Build history of the part. All positions in model axes, mm. Face numbers are marked on the shaded views. A direction names the side the tool comes from. Give positions to 0.01 mm unless a question says otherwise; leave off trailing zeros. Write each loop counter-clockwise with the first axis right and the second up, starting at its lowest first coordinate (ties: lowest second). Pieces come first, ordered by that corner, then holes. Notation, with made-up numbers: M -3,-4.5 L 16,-4.5 A21 ccw 16,11.5 Z; hole C 28,-9 d5. An arc over 180 degrees is marked long. Return JSON: item names as keys, results as strings. Group by question number.
Q1. Band-saw the part on A-A, the plane y = 1. Give the cut face in (x, z).
Q2. Wall check: probe 1 along Y at (x, z) = (1.4, 5.25); probe 2 along Z at (x, y) = (1.95, 5.25); probe 3 along Z at (x, y) = (0.2, 3). Give the ranges that are in metal, low to high.
Q3. Band-saw the part on B-B, the plane z = 2.75. Give the cut face in (x, y), then the cut area to 3 significant figures.
Q4. Pull direction Z, two halves, no side cores. Call the marked faces 1, 2 and 3: +Z half, -Z half, draft (parallel to the pull), parting line (faces both ways), or undercut.
Q5. Flat gauge pins, fed straight in: pin 1 Ø1.5 at (x, y) = (2, 1) entering from -Z; pin 2 Ø1.5 at (x, y) = (0.5, 0) entering from +Z; pin 3 Ø4 at (y, z) = (0, -0.5) entering from -X. Where does each tip first touch, or does it go through?
Q6. Tool access for the marked faces 4 and 5: list every direction of +Z, -Z, +X, -X, +Y, -Y with a clear straight run to the whole face (end or side of a thin tool).
Q7. Band-saw the part on D-D, the plane y = 13.5. Give the cut face in (x, z).
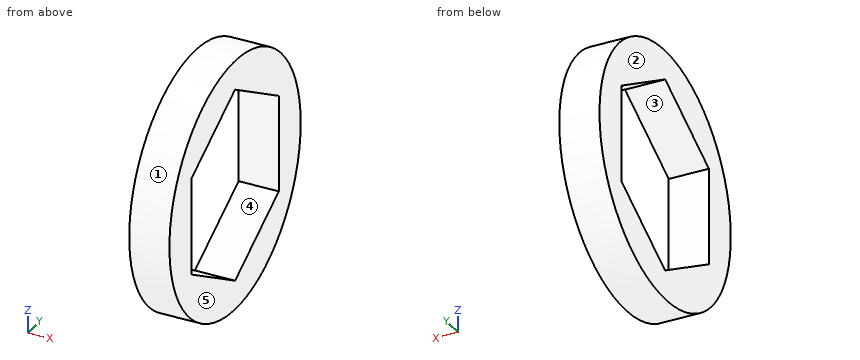
Autodesk Inventor part; units mm, degrees
ref_plane "YZ Plane" through (0, 0, 0) normal (1, 0, 0) x (0, 1, 0)
ref_plane "XZ Plane" through (0, 0, 0) normal (0, 1, 0) x (-1, 0, 0)
ref_plane "XY Plane" through (0, 0, 0) normal (0, 0, 1) x (1, 0, 0)
sketch "Sketch1" plane through (0, 0, 0) normal (1, 0, 0) x (0, 1, 0)
  circle A0 centre (5.9226, 5.0314) radius 9.525
  line L0 (5.9226, 5.0314) -> (12.2726, 5.0314) construction
  line L1 (12.2726, 1.3724) -> (5.9287, -2.2974)
  line L2 (5.9287, -2.2974) -> (-0.4213, 1.3617)
  line L3 (-0.4213, 1.3617) -> (-0.4274, 8.6905)
  line L4 (-0.4274, 8.6905) -> (5.9164, 12.3602)
  line L5 (5.9164, 12.3602) -> (12.2664, 8.7012)
  line L6 (12.2664, 8.7012) -> (12.2726, 1.3724)
  point P0 (0, 0)
  dimension "d0" = 19.05
extrude "Extrusion1" add sketch "Sketch1" along normal blind 3.0226
properties part number "3D Model Spacer"
From the geometry:
{
 "1": {"outline": "M 0,-3.12 L 3.02,-3.12 L 3.02,0.54 L 0,0.54 Z; M 0,9.52 L 3.02,9.52 L 3.02,13.19 L 0,13.19 Z"},
 "2": {"probe 1": "y = -3.6 to -0.42, 12.27 to 15.45", "probe 2": "z = -4.47 to -1.91, 11.97 to 14.53", "probe 3": "z = -4.03 to -0.61, 10.67 to 14.1"},
 "3": {"outline": "M 0,-3.33 L 3.02,-3.33 L 3.02,-0.42 L 0,-0.42 Z; M 0,12.27 L 3.02,12.27 L 3.02,15.17 L 0,15.17 Z", "area": "17.5 mm^2"},
 "4": {"face 1": "parting line", "face 2": "draft", "face 3": "undercut"},
 "5": {"pin 1": "stops at z = -3.53", "pin 2": "stops at z = 13.03", "pin 3": "stops at x = 0"},
 "6": {"face 4": "+X, -X", "face 5": "+Z, -Z, +X, +Y, -Y"},
 "7": {"outline": "M 0,-0.74 L 3.02,-0.74 L 3.02,10.8 L 0,10.8 Z"}
}
